from build123d import *

# Parameters (mm, degrees)
CROQUIS1_W              = 50
CROQUIS1_H              = 50
SALIENTE_EXTRUIR1_DEPTH = 1.3
CROQUIS2_W              = 33.5
CROQUIS2_H              = 5
SALIENTE_EXTRUIR2_DEPTH = 11.1
CROQUIS3_W              = 14.6
CROQUIS3_H              = 9
SALIENTE_EXTRUIR3_DEPTH = 10.9
CROQUIS4_R              = 6.25
SALIENTE_EXTRUIR4_DEPTH = 15.8
CROQUIS5_W              = 13.1
CROQUIS5_H              = 2.6
CROQUIS5_W_2            = 20.8
CROQUIS5_W_3            = 5.5
CROQUIS5_W_4            = 2.6
CROQUIS5_H_2            = 8
CROQUIS5_H_3            = 5.5
SALIENTE_EXTRUIR5_DEPTH = 16.4


with BuildPart() as part:
    # Croquis1 → Saliente-Extruir1 (new body)
    with BuildSketch(Plane.XY):
        with Locations((25, -25)):
            Rectangle(CROQUIS1_W, CROQUIS1_H)
    extrude(amount=SALIENTE_EXTRUIR1_DEPTH)

    # Croquis2 → Saliente-Extruir2 (add)
    with BuildSketch(Plane(origin=(0, 0, 0), x_dir=(-1, 0, 0), z_dir=(0, 0, -1))):
        with Locations((-19.45, -3.7)):
            Rectangle(CROQUIS2_W, CROQUIS2_H)
    extrude(amount=SALIENTE_EXTRUIR2_DEPTH)

    # Croquis3 → Saliente-Extruir3 (add)
    with BuildSketch(Plane.XY.offset(1.3)):
        with Locations((2.7, -42)):
            Rectangle(CROQUIS3_W, CROQUIS3_H)
    extrude(amount=SALIENTE_EXTRUIR3_DEPTH)

    # Croquis4 → Saliente-Extruir4 (add)
    with BuildSketch(Plane.XY.offset(1.3)):
        with Locations((18.25, -41.15)):
            Circle(CROQUIS4_R)
    extrude(amount=SALIENTE_EXTRUIR4_DEPTH)

    # Croquis5 → Saliente-Extruir5 (add)
    with BuildSketch(Plane.XY.offset(1.3)):
        with Locations((40.95, -18.6)):
            Rectangle(CROQUIS5_W, CROQUIS5_H)
        with Locations((22, -18.6)):
            Rectangle(CROQUIS5_W_2, CROQUIS5_H)
        with Locations((6.65, -18.6)):
            Rectangle(CROQUIS5_W_3, CROQUIS5_H)
        with Locations((3.3, -31)):
            Rectangle(CROQUIS5_W_4, CROQUIS5_H_2)
        with Locations((18.8, -29.75)):
            Rectangle(CROQUIS5_W_4, CROQUIS5_H_3)
    extrude(amount=SALIENTE_EXTRUIR5_DEPTH)


solid = part.part
Design review of the part built by this model. Coordinates are the model's own, in mm. A direction names the side the tool comes from. Round coordinates to 2 decimals unless told otherwise and drop trailing zeros. Loops run counter-clockwise (first coordinate to the right, second up) from the corner with the lowest first, then second, coordinate; pieces in that order, holes last. Notation, with made-up numbers: (4, -28.5) -> (43, -28.5) arc R13 cw to (43, -12.5) -> close; hole circle Ø10 at (33.5, 86.25). An arc over 180 degrees is marked (long way). Use one line per item in the form item = value. Start each with the question number.
Q1. We need section C-C on x = 7.5. Give the boundary of the cut face in (y, z), then the cut area to 3 significant figures.
Q2. Wall thickness on line 1 along X through (y, z) = (-31.5, 5.5); line 2 along Z through (x, y) = (46, -7); line 3 along Y through (x, z) = (7, 10): over which ranges is each line inside the solid? List them lowest first. Write a range as [from, to].
Q3. Machinability: for faces 1 (the face through (2.7, -4, -5)), 2 (the face through (20, -6.2, -5)), 3 (the face through (20, -1.2, -5)), 4 (the face through (3, -35, 9)), which of the approach directions +Z, -Z, +X, -X, +Y, -Y give a long, thin tool a straight path to every point of the face, cutting with its end or side? Answer none if there is none.
Q4. We need section A-A on x = 18.25. Give the boundary of the cut face in (y, z), then the cut area to 3 significant figures.
Q5. Draft analysis for pull direction Y (two halves, no side actions). For faces 5 (the face through (7, -19.9, 9)), 6 (the face through (11.6, -19, 9)), 7 (the face through (7, -17.3, 9)), state which applies: +Y half, -Y half, draft (parallel to the pull), parting line (faces both ways), or undercut.
Q6. For pin 1 Ø1.3 at (y, z) = (-19, 12.5) entering from +X; pin 2 Ø3 at (x, z) = (6, 9) entering from -Y; pin 3 Ø2.5 at (x, y) = (-2.5, -42) entering from -Z, all flat-tipped, find the tip position at first contact; note any pin that passes through.
Q7. We need section D-D on z = -5.5. Give the boundary of the cut face in (x, y).
Q8. We need section B-B on y = -5. Give the boundary of the cut face in (x, z).
Calculated:
q1.outline = (-50, 0) -> (-6.2, 0) -> (-6.2, -11.1) -> (-1.2, -11.1) -> (-1.2, 0) -> (0, 0) -> (0, 1.3) -> (-17.3, 1.3) -> (-17.3, 17.7) -> (-19.9, 17.7) -> (-19.9, 1.3) -> (-37.5, 1.3) -> (-37.5, 12.2) -> (-46.5, 12.2) -> (-46.5, 1.3) -> (-50, 1.3) -> close
q1.area = 261 mm²
q2.line_1 = [2, 4.6], [17.5, 20.1]
q2.line_2 = [0, 1.3]
q2.line_3 = [-46.5, -37.5], [-19.9, -17.3]
q3.face_1 = -Z, -X, +Y, -Y
q3.face_2 = -Z, +X, -X, -Y
q3.face_3 = -Z, +X, -X, +Y
q3.face_4 = +Z, -X
q4.outline = (-50, 0) -> (-6.2, 0) -> (-6.2, -11.1) -> (-1.2, -11.1) -> (-1.2, 0) -> (0, 0) -> (0, 1.3) -> (-17.3, 1.3) -> (-17.3, 17.7) -> (-19.9, 17.7) -> (-19.9, 1.3) -> (-27, 1.3) -> (-27, 17.7) -> (-32.5, 17.7) -> (-32.5, 1.3) -> (-34.9, 1.3) -> (-34.9, 17.1) -> (-47.4, 17.1) -> (-47.4, 1.3) -> (-50, 1.3) -> close
q4.area = 451 mm²
q5.face_5 = undercut
q5.face_6 = draft
q5.face_7 = +Y half
q6.pin_1 = 47.5
q6.pin_2 = -46.5
q6.pin_3 = 1.3
q7.outline = (2.7, -6.2) -> (36.2, -6.2) -> (36.2, -1.2) -> (2.7, -1.2) -> close
q8.outline = (0, 0) -> (2.7, 0) -> (2.7, -11.1) -> (36.2, -11.1) -> (36.2, 0) -> (50, 0) -> (50, 1.3) -> (0, 1.3) -> close
